Verification items for this drawing (mm, ordinates from the low corner). A direction names the side the tool comes from. Give positions to 0.01 mm unless a question says otherwise; leave off trailing zeros. Write each loop counter-clockwise with the first axis right and the second up, starting at its lowest first coordinate (ties: lowest second). Pieces come first, ordered by that corner, then holes. Notation, with made-up numbers: (-33, 53.5) -> (24, 53.5) arc R22 cw to (24, 62.5) -> close; hole circle Ø11 at (17, 25.5). An arc over 180 degrees is marked (long way). Use one line per item in the form item = value. Start each with the question number.
(1) Set-up check for the marked faces 1, 2 and 3: record each of +Z, -Z, +X, -X, +Y, -Y from which the full face is reachable in a straight line by a thin tool's end or side.
(2) Section check C-C, the plane z = 32. Record the cut outline in (x, y), plus the area to 3 significant figures.
(3) Scan lines: L1, parallel to Z at x = 13.25, y = 13; L2, parallel to Z at x = 11.25, y = 19.5; L3, parallel to Y at x = 14, z = 25.5. Record each from-to range of solid material in increasing order.
(4) Depth check by flat-ended pin: pin 1 Ø2 at (x, z) = (5, 17.5) entering from +Y; pin 2 Ø8 at (y, z) = (14, 33) entering from -X; pin 3 Ø7 at (x, y) = (16, 11.5) entering from -Z. Enter the tip coordinate at first touch or a pass-through.
(5) Section check B-B, the plane y = 14. Record the cut outline in (x, z), plus the area to 3 significant figures.
(6) Release check for a two-part mould opening along X. For the marked faces 4, 5 and 6 record: pulls with the +X half, pulls with the -X half, needs draft (parallel to the pull), parting line crosses it, or undercut.
(7) Section check D-D, the plane z = 24.5. Record the cut outline in (x, y).
(8) Section check A-A, the plane x = 14. Record the cut outline in (y, z).
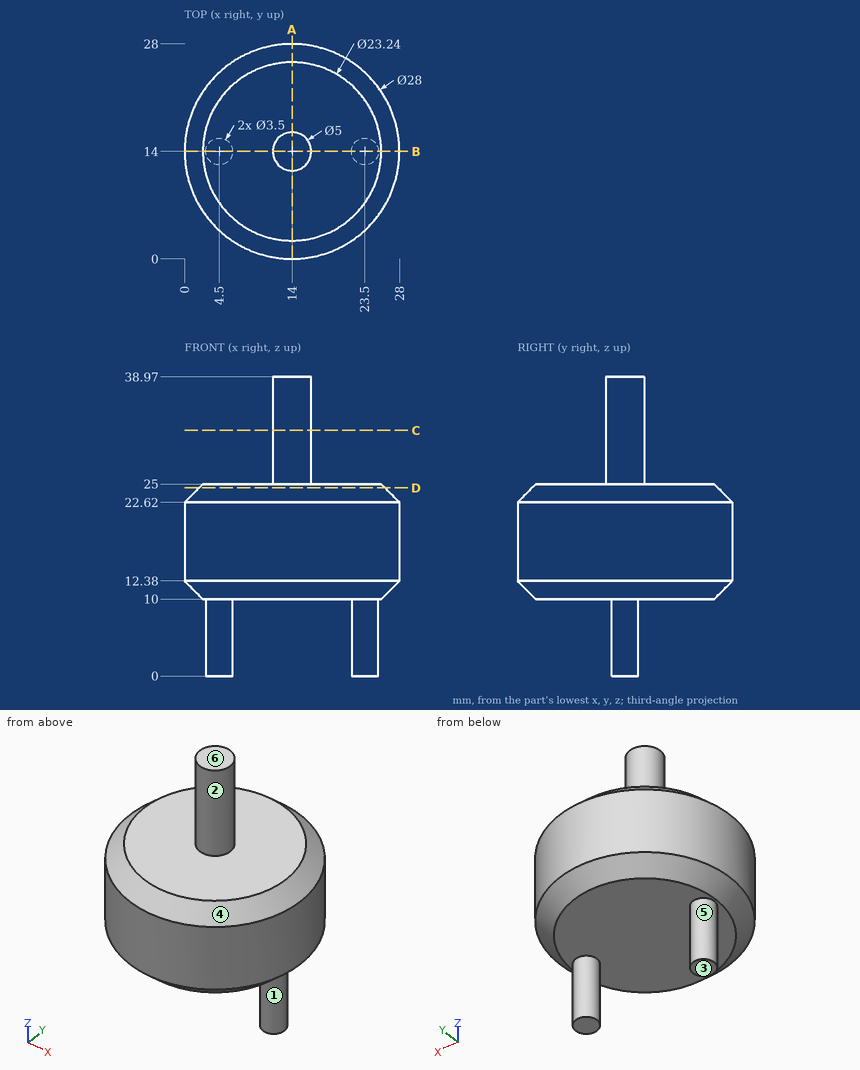
Completed:
q1.face_1 = -Z
q1.face_2 = +Z
q1.face_3 = -Z, +X, -X, +Y, -Y
q2.outline = circle Ø5 at (14, 14)
q2.area = 19.6 mm²
q3.L1 = 10 to 38.97
q3.L2 = 10 to 25
q3.L3 = 11.5 to 16.5
q4.pin_1 = 25.49
q4.pin_2 = 11.5
q4.pin_3 = 10
q5.outline = (0, 12.38) -> (2.38, 10) -> (2.75, 10) -> (2.75, 0) -> (6.25, 0) -> (6.25, 10) -> (21.75, 10) -> (21.75, 0) -> (25.25, 0) -> (25.25, 10) -> (25.62, 10) -> (28, 12.38) -> (28, 22.62) -> (25.62, 25) -> (16.5, 25) -> (16.5, 38.97) -> (11.5, 38.97) -> (11.5, 25) -> (2.38, 25) -> (0, 22.62) -> close
q5.area = 549 mm²
q6.face_4 = parting line crosses it
q6.face_5 = undercut
q6.face_6 = needs draft
q7.outline = circle Ø24.24 at (14, 14)
q8.outline = (0, 12.38) -> (2.38, 10) -> (25.62, 10) -> (28, 12.38) -> (28, 22.62) -> (25.62, 25) -> (16.5, 25) -> (16.5, 38.97) -> (11.5, 38.97) -> (11.5, 25) -> (2.38, 25) -> (0, 22.62) -> close
